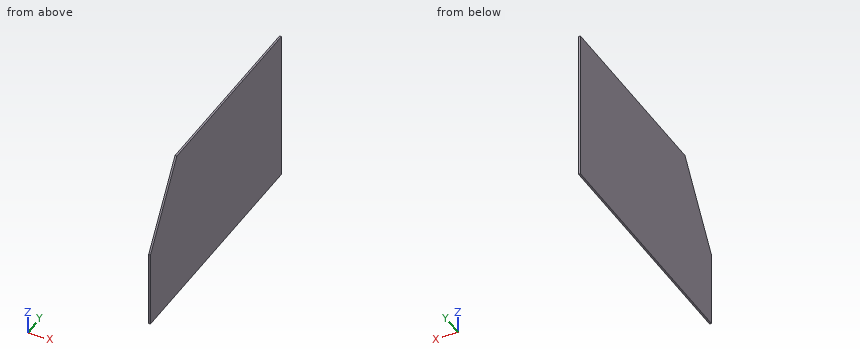
from build123d import *

# Parameters (mm, degrees)
SKETCH1_W           = 3
SKETCH1_H           = 400
BOSS_EXTRUDE1_DEPTH = 255
CUT_EXTRUDE1_DEPTH  = 371.88080499


with BuildPart() as part:
    # Sketch1 → Boss-Extrude1 (new body)
    with BuildSketch(Plane.XY):
        with Locations((-139.199495781, 69.292724577)):
            Rectangle(SKETCH1_W, SKETCH1_H)
    extrude(amount=-BOSS_EXTRUDE1_DEPTH)

    # Sketch2 → Cut-Extrude1 (cut, through all)
    with BuildSketch(Plane.ZY.offset(140.699495781)):
        Polygon((0, -130.707275423), (0, -50), (-127.5, -130.707275423), align=None)
    extrude(amount=-CUT_EXTRUDE1_DEPTH, mode=Mode.SUBTRACT)


solid = part.part
Source: CAD feature listing. Evaluate the final solid. Frame: model axes, mm. Round coordinates to 2 decimals unless told otherwise and drop trailing zeros. Write each loop counter-clockwise with the first axis right and the second up, starting at its lowest first coordinate (ties: lowest second). Pieces come first, ordered by that corner, then holes. Notation, with made-up numbers: (59, 88) - (70, 88) arc R25 ccw to (70, 119) - close; hole circle Ø2 at (88, -35). An arc over 180 degrees is marked (long way). Use CSV: the item, a comma, the result in double quotes. Start each with the question number.
(1) Cut plane C-C, the plane z = -108. Return loops of the section in (x, y).
(2) Material intervals for probe 1 along Y at (x, z) = (-140.2, -25); probe 2 along Y at (x, z) = (-140.35, -34.5); probe 3 along Z at (x, y) = (-138.5, -72), sorted ascending. Write a range as [from, to].
(3) Cut plane B-B, the plane y = -59. Return loops of the section in (x, z), and give its area (3 significant figures).
(4) Cut plane A-A, the plane x = -138.9. Return loops of the section in (y, z), and give its area (3 significant figures).
Geometry says:
1,outline,"(-140.7, -118.36) - (-137.7, -118.36) - (-137.7, 269.29) - (-140.7, 269.29) - close"
2,probe 1,"[-65.82, 269.29]"
2,probe 2,"[-71.84, 269.29]"
2,probe 3,"[-255, -34.76]"
3,outline,"(-140.7, -255) - (-137.7, -255) - (-137.7, -14.22) - (-140.7, -14.22) - close"
3,area,"722 mm²"
4,outline,"(-130.71, -255) - (269.29, -255) - (269.29, 0) - (-50, 0) - (-130.71, -127.5) - close"
4,area,"96,900 mm²"
